from build123d import *

# Parameters (mm, degrees)
SKETCH1_W            = 100
SKETCH1_H            = 160
BOSS_EXTRUDE1_DEPTH  = 3
M3_CLEARANCE_HOLE1_D = 3.4
M3_CLEARANCE_HOLE2_D = 3.4
CUT_EXTRUDE1_REACH   = 96.387
SKETCH6_W            = 28
SKETCH6_H            = 10.5
SKETCH6_W_2          = 20
SKETCH6_H_2          = 7
FILLET1_R            = 5
FILLET2_R            = 2


with BuildPart() as part:
    # Sketch1 → Boss-Extrude1 (new body)
    with BuildSketch(Plane(origin=(0, 0, 0), x_dir=(1, 0, 0), z_dir=(0, 1, 0))):
        Rectangle(SKETCH1_W, SKETCH1_H)
    extrude(amount=BOSS_EXTRUDE1_DEPTH)

    # M3 Clearance Hole1 (through all)
    with Locations(Plane(origin=(0, 3, 0), x_dir=(1, 0, 0), z_dir=(0, 1, 0))):
        with Locations((-35, 62), (-35, 69), (-42, 62), (-35, 55), (-28, 62), (35, 69), (28, 62), (35, 62), (42, 62), (35, 55), (-35, -62), (-42, -62), (-35, -55), (-28, -62), (-35, -69), (35, -62), (35, -55), (28, -62), (42, -62), (35, -69)):
            Hole(M3_CLEARANCE_HOLE1_D / 2)

    # M3 Clearance Hole2 (through all)
    with Locations(Plane(origin=(0, 3, 0), x_dir=(1, 0, 0), z_dir=(0, 1, 0))):
        with Locations((0, 0), (0, 7), (7, 0), (0, -7), (-7, 0)):
            Hole(M3_CLEARANCE_HOLE2_D / 2)

    # Sketch6 → Cut-Extrude1 (cut, up to next)
    with BuildSketch(Plane(origin=(0, 3, 0), x_dir=(1, 0, 0), z_dir=(0, 1, 0)), mode=Mode.PRIVATE) as cut_extrude1_sk1:
        with Locations((0, -60)):
            Rectangle(SKETCH6_W, SKETCH6_H)
    cut_extrude1_tool1 = extrude(cut_extrude1_sk1.sketch, amount=-CUT_EXTRUDE1_REACH, mode=Mode.PRIVATE) & part.part
    # Sketch6 → Cut-Extrude1 (cut, up to next)
    with BuildSketch(Plane(origin=(0, 3, 0), x_dir=(1, 0, 0), z_dir=(0, 1, 0)), mode=Mode.PRIVATE) as cut_extrude1_sk2:
        with Locations((0, -43)):
            Rectangle(SKETCH6_W_2, SKETCH6_H_2)
    cut_extrude1_tool2 = extrude(cut_extrude1_sk2.sketch, amount=-CUT_EXTRUDE1_REACH, mode=Mode.PRIVATE) & part.part
    add(cut_extrude1_tool1.solids().sort_by_distance((0, 3, 60))[0], mode=Mode.SUBTRACT)
    add(cut_extrude1_tool2.solids().sort_by_distance((0, 3, 43))[0], mode=Mode.SUBTRACT)

    # Fillet1
    fillet1_edges = [part.edges().sort_by_distance(p)[0] for p in [
        (50, 1.5, 80),
        (-50, 1.5, 80),
        (-50, 1.5, -80),
        (50, 1.5, -80),
    ]]
    fillet(fillet1_edges, radius=FILLET1_R)

    # Fillet2
    fillet2_edges = [part.edges().sort_by_distance(p)[0] for p in [
        (-14, 1.5, 65.25),
        (-14, 1.5, 54.75),
        (14, 1.5, 54.75),
        (14, 1.5, 65.25),
        (10, 1.5, 39.5),
        (10, 1.5, 46.5),
        (-10, 1.5, 46.5),
        (-10, 1.5, 39.5),
    ]]
    fillet(fillet2_edges, radius=FILLET2_R)


solid = part.part
Geometry check sheet. Reference: the model listing, model coordinates, mm. A direction names the side the tool comes from. Give positions to 0.01 mm unless a question says otherwise; leave off trailing zeros. Order: outer loops, then holes, each group sorted by start corner. A loop starts at its lowest first (then second) coordinate and runs counter-clockwise, first axis right, second up. Notation, with made-up numbers: (23, -9) - (28, -9) arc R38 ccw to (28, 29) - close; hole circle Ø9 at (-30, -35.5). An arc over 180 degrees is marked (long way). Answer as a JSON object with one key per item and string values.
(1) Material ranges on line 1 (Z direction, x = -28, y = 1.4); line 2 (Z direction, x = -7, y = 0.9); line 3 (Z direction, x = 3, y = 0.25), recorded low to high.
Report:
{"line 1": "-80 to -63.7, -60.3 to 60.3, 63.7 to 80", "line 2": "-80 to -1.7, 1.7 to 39.5, 46.5 to 54.75, 65.25 to 80", "line 3": "-80 to 39.5, 46.5 to 54.75, 65.25 to 80"}
(2) Cross-section at D-D (z = -7). Record the cut outline in (x, y), then the cut area to 3 significant figures.
Report:
{"outline": "(-50, 0) - (-1.7, 0) - (-1.7, 3) - (-50, 3) - close; (1.7, 0) - (50, 0) - (50, 3) - (1.7, 3) - close", "area": "290 mm^2"}
(3) Cross-section at C-C (z = -69). Record the cut outline in (x, y), then the cut area to 3 significant figures.
Report:
{"outline": "(-50, 0) - (-36.7, 0) - (-36.7, 3) - (-50, 3) - close; (-33.3, 0) - (33.3, 0) - (33.3, 3) - (-33.3, 3) - close; (36.7, 0) - (50, 0) - (50, 3) - (36.7, 3) - close", "area": "280 mm^2"}
(4) Cross-section at B-B (x = 28). Record the cut outline in (y, z).
Report:
{"outline": "(0, -80) - (3, -80) - (3, -63.7) - (0, -63.7) - close; (0, -60.3) - (3, -60.3) - (3, 60.3) - (0, 60.3) - close; (0, 63.7) - (3, 63.7) - (3, 80) - (0, 80) - close"}
(5) Depth check by flat-ended pin: pin 1 Ø2 at (x, z) = (-28, -62) entering from +Y. Enter the tip coordinate at first touch or a pass-through.
Report:
{"pin 1": "through"}
(6) Draft check along X on faces 1 (the flat face through (-1, 1, -80)), 2 (the flat face through (50, 1, 1)), 3 (the cylindrical face through (27.086, 1.479, 60.567)). Enter one of: released by +X, released by -X, zero draft, split by the parting line, or undercut.
Report:
{"face 1": "zero draft", "face 2": "released by +X", "face 3": "undercut"}
(7) Cross-section at A-A (x = 0). Record the cut outline in (y, z), then the cut area to 3 significant figures.
Report:
{"outline": "(0, -80) - (3, -80) - (3, -8.7) - (0, -8.7) - close; (0, -5.3) - (3, -5.3) - (3, -1.7) - (0, -1.7) - close; (0, 1.7) - (3, 1.7) - (3, 5.3) - (0, 5.3) - close; (0, 8.7) - (3, 8.7) - (3, 39.5) - (0, 39.5) - close; (0, 46.5) - (3, 46.5) - (3, 54.75) - (0, 54.75) - close; (0, 65.25) - (3, 65.25) - (3, 80) - (0, 80) - close", "area": "397 mm^2"}
(8) Tool access check on faces 4 (the flat face through (-1, 1, 80)), 5 (the flat face through (10, 2, 43)). Record the directions out of +Z, -Z, +X, -X, +Y, -Y that give a thin tool (end or side, any length) a straight path to the whole face; none if there is none.
Report:
{"face 4": "+Z, +X, -X, +Y, -Y", "face 5": "+Y, -Y"}
